Work out the finished part from the listing and answer in its coordinate system (mm). A direction names the side the tool comes from. Give positions to 0.01 mm unless a question says otherwise; leave off trailing zeros. Loops run counter-clockwise (first coordinate to the right, second up) from the corner with the lowest first, then second, coordinate; pieces in that order, holes last. Notation, with made-up numbers: M 1.25,25 L 15.25,25 A15 cw 15.25,51 Z; hole C -21,-29.75 d5. An arc over 180 degrees is marked long. Write item = value, one per line. Start each with the question number.
1. Section D-D on x = 18 is taken. Determine the outline of the cut face in (y, z).
2. Section A-A on x = 0 is taken. Determine the outline of the cut face in (y, z).
3. For faces 1 (the face through (3.47, 4.54, -15.62)), 2 (the face through (-22, 5, 0)), 3 (the face through (-12.15, 1.479, 18.965)), 4 (the face through (0, 5, -22)), 5 (the face through (21.14, 5.52, 21.1)), determine the directions among +Z, -Z, +X, -X, +Y, -Y from which every point of the face is accessible in a straight line to the end or side of a thin tool.
4. Consider L1, parallel to Z at x = -16.5, y = 4.75; L2, parallel to Z at x = 16.5, y = 3.9; L3, parallel to X at y = 2.5, z = -12. Determine where each line is inside the solid, lowest interval first. Write a range as [from, to].
5. Section C-C on y = 6.25 is taken. Determine the outline of the cut face in (x, z).
6. The mould has two halves that part along X. Classify faces 6 (the face through (-21.1, 5.52, 21.14)), 7 (the face through (-20.85, 1.479, 14.035)), 8 (the face through (16, 1, 11.5)), 9 (the face through (0, 5, 22)): released by +X, released by -X, zero draft, split by the parting line, or undercut.
7. A flat-ended cylindrical pin translates along its axis: pin 1 Ø3 at (x, z) = (-17.5, 15) entering from -Y. Find the tip coordinate at first contact, or state that the pin passes through.
8. Section B-B on z = 0 is taken. Determine the outline of the cut face in (x, y).
```python
from build123d import *

# Parameters (mm, degrees)
F0_W      = 50
F0_H      = 50
F1_DEPTH  = 4
F2_W      = 44
F2_H      = 44
F3_DEPTH  = 3
F4_R      = 3
F4_R_2    = 7.5
F5_DEPTH  = 25
F7_DEPTH  = 3
F8_R      = 12
F9_DEPTH  = 5
F10_R     = 16
F11_DEPTH = 5
F12_R     = 12.5
F13_DEPTH = 2.001
F14_R     = 3


with BuildPart() as f1:
    # F0 (on Front) → F1 (new body)
    with BuildSketch(Plane.XZ):
        Rectangle(F0_W, F0_H)
    extrude(amount=-F1_DEPTH)

    # F2 (on face) → F3 (join)
    with BuildSketch(Plane(origin=(0, 4, 0), x_dir=(-1, 0, 0), z_dir=(0, 1, 0))):
        Rectangle(F2_W, F2_H)
    extrude(amount=F3_DEPTH)

    # F4 (on face) → F5 (cut)
    with BuildSketch(Plane(origin=(0, 7, 0), x_dir=(-1, 0, 0), z_dir=(0, 1, 0))):
        with Locations((-16.5, 16.5)):
            Circle(F4_R)
        with Locations((16.5, 16.5)):
            Circle(F4_R)
        with Locations((16.5, -16.5)):
            Circle(F4_R)
        with Locations((-16.5, -16.5)):
            Circle(F4_R)
        Circle(F4_R_2)
    extrude(amount=-F5_DEPTH, mode=Mode.SUBTRACT)

    # F6 (on face) → F7 (cut)
    with BuildSketch(Plane.XZ):
        Polygon((-19.386751, 11.5), (-13.613249, 11.5), (-10.726497, 16.5), (-13.613249, 21.5), (-19.386751, 21.5), (-22.273503, 16.5), align=None)
        Polygon((19.386751, 21.5), (13.613249, 21.5), (10.726497, 16.5), (13.613249, 11.5), (19.386751, 11.5), (22.273503, 16.5), align=None)
        Polygon((13.613249, -21.5), (19.386751, -21.5), (22.273503, -16.5), (19.386751, -11.5), (13.613249, -11.5), (10.726497, -16.5), align=None)
        Polygon((-19.386751, -21.5), (-13.613249, -21.5), (-10.726497, -16.5), (-13.613249, -11.5), (-19.386751, -11.5), (-22.273503, -16.5), align=None)
    extrude(amount=-F7_DEPTH, mode=Mode.SUBTRACT)

    # F8 (on face) → F9 (cut)
    with BuildSketch(Plane(origin=(0, 7, 0), x_dir=(-1, 0, 0), z_dir=(0, 1, 0))):
        Circle(F8_R)
    extrude(amount=-F9_DEPTH, mode=Mode.SUBTRACT)

    # F10 (on face) → F11 (cut)
    with BuildSketch(Plane(origin=(0, 7, 0), x_dir=(-1, 0, 0), z_dir=(0, 1, 0))):
        Circle(F10_R)
    extrude(amount=-F11_DEPTH, mode=Mode.SUBTRACT)

    # F12 (on face) → F13 (cut, through all)
    with BuildSketch(Plane(origin=(0, 2, 0), x_dir=(-1, 0, 0), z_dir=(0, 1, 0))):
        Circle(F12_R)
    extrude(amount=-F13_DEPTH, mode=Mode.SUBTRACT)

    # F14
    f14_edges = [f1.edges().sort_by_distance(p)[0] for p in [
        (22, 5.5, 22),
        (-22, 5.5, 22),
        (-22, 5.5, -22),
        (22, 5.5, -22),
    ]]
    fillet(f14_edges, radius=F14_R)


solid = f1.part
```
Verdict:
q1.outline = M 0,-25 L 4,-25 L 4,-22 L 7,-22 L 7,-19.1 L 3,-19.1 L 3,-21.5 L 0,-21.5 Z; M 0,-11.5 L 3,-11.5 L 3,-13.9 L 7,-13.9 L 7,13.9 L 3,13.9 L 3,11.5 L 0,11.5 Z; M 0,21.5 L 3,21.5 L 3,19.1 L 7,19.1 L 7,22 L 4,22 L 4,25 L 0,25 Z
q2.outline = M 0,-25 L 4,-25 L 4,-22 L 7,-22 L 7,-16 L 2,-16 L 2,-12.5 L 0,-12.5 Z; M 0,12.5 L 2,12.5 L 2,16 L 7,16 L 7,22 L 4,22 L 4,25 L 0,25 Z
q3.face_1 = +Y
q3.face_2 = +Z, -Z, -X, +Y
q3.face_3 = -Y
q3.face_4 = -Z, +X, -X, +Y
q3.face_5 = +Z, +X, +Y
q4.L1 = [-22, -19.5], [-13.5, 13.5], [19.5, 22]
q4.L2 = [-25, -19.5], [-13.5, 13.5], [19.5, 25]
q4.L3 = [-25, -19.68], [-13.32, -10.58], [10.58, 13.32], [19.68, 25]
q5.outline = M -22,-19 A3 ccw -19,-22 L 19,-22 A3 ccw 22,-19 L 22,19 A3 ccw 19,22 L -19,22 A3 ccw -22,19 Z; hole C -16.5,-16.5 d6; hole C -16.5,16.5 d6; hole C 0,0 d32; hole C 16.5,-16.5 d6; hole C 16.5,16.5 d6
q6.face_6 = released by -X
q6.face_7 = undercut
q6.face_8 = undercut
q6.face_9 = zero draft
q7.pin_1 = 3
q8.outline = M -25,0 L -12.5,0 L -12.5,2 L -16,2 L -16,7 L -22,7 L -22,4 L -25,4 Z; M 12.5,0 L 25,0 L 25,4 L 22,4 L 22,7 L 16,7 L 16,2 L 12.5,2 Z
